Read the model definition and answer for the solid it produces. Units are mm, in the model's axes. Face numbers are marked on the shaded views. A direction names the side the tool comes from. Round coordinates to 2 decimals unless told otherwise and drop trailing zeros. Order: outer loops, then holes, each group sorted by start corner. A loop starts at its lowest first (then second) coordinate and runs counter-clockwise, first axis right, second up. Notation, with made-up numbers: (43.5, 18.25) -> (57.5, 18.25) arc R29 ccw to (57.5, 57.25) -> close; hole circle Ø8 at (65, 32). An arc over 180 degrees is marked (long way). Answer as a JSON object with one key per item and string values. Group by question number.
Item 1: For the marked faces 5 and 6, determine the directions among +Z, -Z, +X, -X, +Y, -Y from which every point of the face is accessible in a straight line to the end or side of a thin tool.
Item 2: Given P1, Ø1.1, axis at x = -0.5, z = 0.5, coming from the +Y side; P2, Ø4, axis at x = 9, z = 3.5, coming from the -Y side, each flat-ended and moving along its own axis, determine where each tip first touches the part or whether it passes through.
Item 3: The mould has two halves that part along Y. Classify the marked faces 1, 2, 3 and 4: pulls with the +Y half, pulls with the -Y half, needs draft (parallel to the pull), parting line crosses it, or undercut.
Item 4: Consider probe 1 along X at (y, z) = (2.8, -6.5); probe 2 along Z at (x, y) = (3.5, 3.65); probe 3 along Y at (x, z) = (6, -4.75). Determine where each line is inside the solid, lowest interval first. Write a range as from..to.
Item 5: Section D-D, the plane z = 1.25 is taken. Write down the section's boundary in (x, y), plus the area to 3 significant figures.
Item 6: Section C-C, the plane x = 6.25 is taken. Write down the section's boundary in (y, z).
Item 7: Section A-A, the plane y = 3.5 is taken. Write down the section's boundary in (x, z).
Item 8: Section B-B, the plane z = -6 is taken. Write down the section's boundary in (x, y).
from build123d import *

# Parameters (mm, degrees)
SKETCH_2_W           = 10.5
SKETCH_2_H           = 4
EXTRUDE_1_DEPTH      = 1
SKETCH_3_W           = 1
SKETCH_3_H           = 16
EXTRUDE_2_DEPTH      = 2.3
EXTRUDE_2_DEPTH_BACK = 1
SKETCH_4_W           = 12.5
SKETCH_4_H           = 4
EXTRUDE_3_DEPTH      = 1


with BuildPart() as part:
    # 草图2 → 凸台-拉伸1 (new body)
    with BuildSketch(Plane(origin=(0, 0, 0), x_dir=(1, 0, 0), z_dir=(0, 1, 0))):
        with Locations((5.25, 6)):
            Rectangle(SKETCH_2_W, SKETCH_2_H)
        with Locations((5.25, 2)):
            Rectangle(SKETCH_2_W, SKETCH_2_H)
        with Locations((5.25, -2)):
            Rectangle(SKETCH_2_W, SKETCH_2_H)
        with Locations((5.25, -6)):
            Rectangle(SKETCH_2_W, SKETCH_2_H)
    extrude(amount=EXTRUDE_1_DEPTH)

    # 草图3 → 凸台-拉伸2 (add, two sides)
    with BuildSketch(Plane(origin=(0, 1, 0), x_dir=(1, 0, 0), z_dir=(0, 1, 0))) as extrude_2_sk:
        with Locations((11, 0)):
            Rectangle(SKETCH_3_W, SKETCH_3_H)
        with Locations((-0.5, 0)):
            Rectangle(SKETCH_3_W, SKETCH_3_H)
    extrude(amount=EXTRUDE_2_DEPTH)
    extrude(extrude_2_sk.sketch, amount=-EXTRUDE_2_DEPTH_BACK)

    # 草图4 → 凸台-拉伸3 (add)
    with BuildSketch(Plane(origin=(0, 3.3, 0), x_dir=(1, 0, 0), z_dir=(0, 1, 0))):
        with Locations((5.25, 6)):
            Rectangle(SKETCH_4_W, SKETCH_4_H)
        with Locations((5.25, -6)):
            Rectangle(SKETCH_4_W, SKETCH_4_H)
    extrude(amount=EXTRUDE_3_DEPTH)


solid = part.part
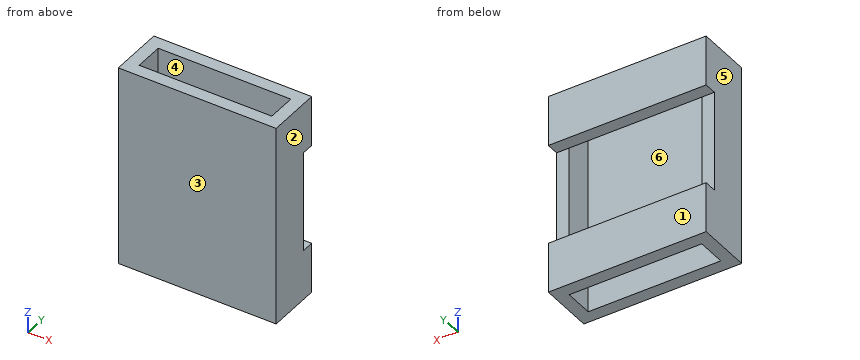
Values found:
{
 "1": {"face 5": "+Z, -Z, -X, +Y, -Y", "face 6": "+Z, -Z"},
 "2": {"P1": "y = 3.3", "P2": "y = 0"},
 "3": {"face 1": "pulls with the +Y half", "face 2": "needs draft", "face 3": "pulls with the -Y half", "face 4": "undercut"},
 "4": {"probe 1": "-1..0, 10.5..11.5", "probe 2": "-8..-4, 4..8", "probe 3": "0..1, 3.3..4.3"},
 "5": {"outline": "(-1, 0) -> (11.5, 0) -> (11.5, 3.3) -> (10.5, 3.3) -> (10.5, 1) -> (0, 1) -> (0, 3.3) -> (-1, 3.3) -> close", "area": "17.1 mm2"},
 "6": {"outline": "(0, -8) -> (1, -8) -> (1, 8) -> (0, 8) -> close; (3.3, -8) -> (4.3, -8) -> (4.3, -4) -> (3.3, -4) -> close; (3.3, 4) -> (4.3, 4) -> (4.3, 8) -> (3.3, 8) -> close"},
 "7": {"outline": "(-1, -8) -> (11.5, -8) -> (11.5, -4) -> (-1, -4) -> close; (-1, 4) -> (11.5, 4) -> (11.5, 8) -> (-1, 8) -> close"},
 "8": {"outline": "(-1, 0) -> (11.5, 0) -> (11.5, 4.3) -> (-1, 4.3) -> close; hole (0, 1) -> (10.5, 1) -> (10.5, 3.3) -> (0, 3.3) -> close"}
}
